from build123d import *

# Parameters (mm, degrees)
SKETCH1_R           = 1
SKETCH1_R_2         = 5
BOSS_EXTRUDE1_DEPTH = 3
FILLET1_R           = 1
FILLET3_R           = 1


with BuildPart() as part:
    # Sketch1 → Boss-Extrude1 (new body)
    with BuildSketch(Plane.ZY.offset(-664.925949728)):
        with BuildLine():
            Line((1323.317943891, 920.63265885), (1328.917943891, 920.63265885))
            Line((1328.917943891, 920.63265885), (1328.917943891, 913.632658853))
            ThreePointArc((1328.917943891, 913.632658853), (1330.968196422, 908.682911384), (1335.917943891, 906.632658853))
            Line((1335.917943891, 906.632658853), (1342.917943891, 906.632658853))
            Line((1342.917943891, 906.632658853), (1342.917943891, 901.03265885))
            Line((1342.917943891, 901.03265885), (1335.917943891, 901.03265885))
            ThreePointArc((1335.917943891, 901.03265885), (1330.968196422, 898.982406318), (1328.917943891, 894.03265885))
            Line((1328.917943891, 894.03265885), (1328.917943891, 887.03265885))
            Line((1328.917943891, 887.03265885), (1323.317943893, 887.03265885))
            Line((1323.317943893, 887.03265885), (1323.317943893, 894.03265885))
            ThreePointArc((1323.317943893, 894.03265885), (1321.267691361, 898.982406318), (1316.317943893, 901.03265885))
            Line((1316.317943893, 901.03265885), (1309.317943891, 901.03265885))
            Line((1309.317943891, 901.03265885), (1309.317943891, 906.632658853))
            Line((1309.317943891, 906.632658853), (1316.317943891, 906.632658853))
            ThreePointArc((1316.317943891, 906.632658853), (1321.267691359, 908.682911384), (1323.317943891, 913.632658853))
            Line((1323.317943891, 913.632658853), (1323.317943891, 920.63265885))
        make_face()
        with Locations((1326.117943891, 918.03265885)):
            Circle(SKETCH1_R, mode=Mode.SUBTRACT)
        with Locations((1311.917943891, 903.832658851)):
            Circle(SKETCH1_R, mode=Mode.SUBTRACT)
        with Locations((1340.317943891, 903.832658851)):
            Circle(SKETCH1_R, mode=Mode.SUBTRACT)
        with Locations((1326.117943892, 889.63265885)):
            Circle(SKETCH1_R, mode=Mode.SUBTRACT)
        with Locations((1326.117943891, 903.83265885)):
            Circle(SKETCH1_R_2, mode=Mode.SUBTRACT)
    extrude(amount=BOSS_EXTRUDE1_DEPTH)

    # Fillet1
    fillet1_edges = [part.edges().sort_by_distance(p)[0] for p in [
        (663.425949728, 920.63265885, 1323.317943891),
        (663.425949728, 920.63265885, 1328.917943891),
        (663.425949728, 906.632658853, 1342.917943891),
        (663.425949728, 901.03265885, 1342.917943891),
        (663.425949728, 887.03265885, 1328.917943891),
        (663.425949728, 887.03265885, 1323.317943893),
        (663.425949728, 901.03265885, 1309.317943891),
        (663.425949728, 906.632658853, 1309.317943891),
    ]]
    fillet(fillet1_edges, radius=FILLET1_R)

    # Fillet3
    fillet3_edges = [part.edges().sort_by_distance(p)[0] for p in [
        (661.925949728, 906.632658853, 1313.317943891),
        (664.925949728, 916.632658851, 1328.917943891),
        (664.925949728, 908.682911384, 1330.968196422),
        (664.925949728, 901.03265885, 1338.917943891),
        (664.925949728, 898.982406318, 1330.968196422),
        (664.925949728, 891.03265885, 1323.317943893),
        (664.925949728, 898.982406318, 1321.267691361),
        (664.925949728, 906.632658853, 1313.317943891),
        (664.925949728, 908.682911384, 1321.267691359),
        (661.925949728, 898.982406318, 1321.267691361),
        (661.925949728, 891.03265885, 1323.317943893),
        (661.925949728, 898.982406318, 1330.968196422),
        (661.925949728, 901.03265885, 1338.917943891),
        (661.925949728, 908.682911384, 1330.968196422),
        (661.925949728, 916.632658851, 1328.917943891),
        (664.925949728, 906.632658853, 1338.917943891),
        (661.925949728, 906.632658853, 1338.917943891),
        (664.925949728, 916.632658851, 1323.317943891),
        (664.925949728, 920.63265885, 1326.117943891),
        (664.925949728, 903.832658851, 1342.917943891),
        (664.925949728, 891.03265885, 1328.917943891),
        (664.925949728, 887.03265885, 1326.117943892),
        (664.925949728, 901.03265885, 1313.317943892),
        (664.925949728, 903.832658851, 1309.317943891),
        (664.925949728, 920.339765631, 1328.625050672),
        (664.925949728, 906.339765634, 1309.610837109),
        (664.925949728, 920.339765631, 1323.610837109),
        (664.925949728, 901.325552068, 1309.610837109),
        (664.925949728, 887.325552069, 1323.610837112),
        (664.925949728, 887.325552069, 1328.625050672),
        (664.925949728, 901.325552068, 1342.625050672),
        (664.925949728, 906.339765634, 1342.625050672),
        (661.925949728, 903.832658851, 1342.917943891),
        (661.925949728, 916.632658851, 1323.317943891),
        (661.925949728, 903.832658851, 1309.317943891),
        (661.925949728, 901.03265885, 1313.317943892),
        (661.925949728, 887.03265885, 1326.117943892),
        (661.925949728, 891.03265885, 1328.917943891),
        (661.925949728, 920.63265885, 1326.117943891),
        (661.925949728, 920.339765631, 1328.625050672),
        (661.925949728, 906.339765634, 1309.610837109),
        (661.925949728, 920.339765631, 1323.610837109),
        (661.925949728, 901.325552068, 1309.610837109),
        (661.925949728, 887.325552069, 1323.610837112),
        (661.925949728, 887.325552069, 1328.625050672),
        (661.925949728, 901.325552068, 1342.625050672),
        (661.925949728, 906.339765634, 1342.625050672),
        (661.925949728, 908.682911384, 1321.267691359),
    ]]
    fillet(fillet3_edges, radius=FILLET3_R)


solid = part.part
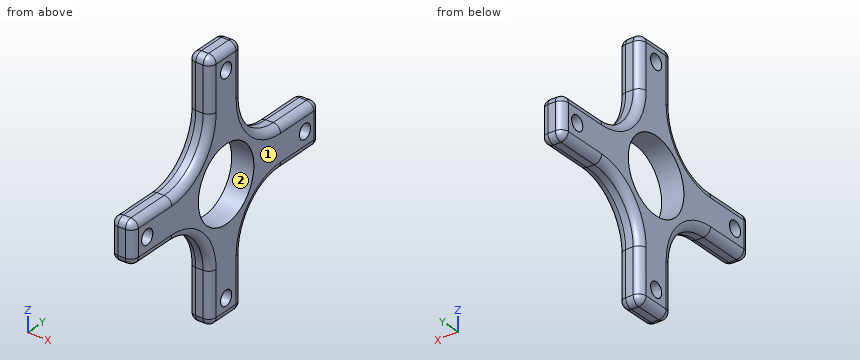
Work out the finished part from the listing and answer in its coordinate system (mm). Face numbers are marked on the shaded views. Coordinates: 2 decimals unless noted, no trailing zeros. Write each loop counter-clockwise with the first axis right and the second up, starting at its lowest first coordinate (ties: lowest second). Pieces come first, ordered by that corner, then holes.
1. The part is cut by section C-C, the plane x = 664.45. State how many separate pieces and enclosed holes the cut face has, and give its area (3 significant figures).
Results list:
separate pieces: 1
enclosed holes: 5
area: 277 mm2
2. For a pull along Y with two mould halves and no side action, classify the marked faces 1 and 2 as +Y half, -Y half, draft (parallel to the pull), parting line (faces both ways), or undercut.
Results list:
face 1: draft
face 2: undercut
3. The part is cut by section B-B, the plane y = 892.5. Write down the section's boundary in (x, z).
Results list:
outline: (661.93, 1324.32) arc R1 ccw to (662.93, 1323.32) - (663.93, 1323.32) arc R1 ccw to (664.93, 1324.32) - (664.93, 1327.92) arc R1 ccw to (663.93, 1328.92) - (662.93, 1328.92) arc R1 ccw to (661.93, 1327.92) - close
4. Consider line 1 along Z through (x, y) = (664.3, 903); line 2 along Z through (x, y) = (663.65, 903.5); line 3 along Y through (x, z) = (664.05, 1326.5). Determine where each line is inside the solid, lowest interval first.
Results list:
line 1: z = 1309.39 to 1311.36, 1312.47 to 1321.19, 1331.05 to 1339.76, 1340.87 to 1342.85
line 2: z = 1309.32 to 1310.97, 1312.86 to 1321.13, 1331.11 to 1339.37, 1341.26 to 1342.92
line 3: y = 887.04 to 888.71, 890.56 to 898.85, 908.82 to 917.11, 918.96 to 920.62
5. The part is cut by section A-A, the plane z = 1327.5. Write down the section's boundary in (x, y), and give its area (3 significant figures).
Results list:
outline: (661.93, 888.03) arc R1 ccw to (662.93, 887.03) - (663.93, 887.03) arc R1 ccw to (664.93, 888.03) - (664.93, 899.03) - (661.93, 899.03) - close; (661.93, 908.64) - (664.93, 908.64) - (664.93, 919.63) arc R1 ccw to (663.93, 920.63) - (662.93, 920.63) arc R1 ccw to (661.93, 919.63) - close
area: 71.1 mm2
6. Flat-ended cylindrical pins translate along their axes: pin 1 (0.8 mm diameter, centred on x = 663.5, z = 1313, fed in from -Y); pin 2 (0.8 mm diameter, centred on x = 663.5, z = 1340.5, fed in from +Y); pin 3 (0.8 mm diameter, centred on x = 663.5, y = 918, fed in from +Z). Find the tip coordinate at first contact, or state that the pin passes through.
Results list:
pin 1: stops at y = 901.03
pin 2: stops at y = 906.63
pin 3: stops at z = 1328.92
7. The part is cut by section D-D, the plane z = 1315. Write down the section's boundary in (x, y).
Results list:
outline: (661.93, 902.03) arc R1 ccw to (662.93, 901.03) - (663.93, 901.03) arc R1 ccw to (664.93, 902.03) - (664.93, 905.63) arc R1 ccw to (663.93, 906.63) - (662.93, 906.63) arc R1 ccw to (661.93, 905.63) - close
